Can you work these out from the model? Positions are in its coordinate system, mm. Face numbers are marked on the shaded views. A direction names the side the tool comes from. Round coordinates to 2 decimals unless told otherwise and drop trailing zeros. Order: outer loops, then holes, each group sorted by start corner. A loop starts at its lowest first (then second) coordinate and runs counter-clockwise, first axis right, second up. Notation, with made-up numbers: (-23.75, 17) -> (13.25, 17) arc R23 cw to (13.25, 49) -> close; hole circle Ø4 at (44, -23.75). An arc over 180 degrees is marked (long way). Use a Markdown table: item, result. Add a question column.
Q1. If we section it at A-A on y = 13: List the corners of the cut face in (x, z) for me, plus the area to 3 significant figures.
Q2. I need wall thicknesses on line 1 along X through (y, z) = (33, 6.8); line 2 along Y through (x, z) = (23, 7.05); line 3 along Y through (x, z) = (-11.5, 1.5). Which ranges of each line are inside material? Lowest first, please. Write a range as [from, to].
Q3. For the marked faces 1, 2 and 3, which set-ups out of +Z, -Z, +X, -X, +Y, -Y let a thin tool reach every point of the face, with its end or its side?
Q4. If we section it at B-B on x = -17: List the corners of the cut face in (y, z) for me.
Q5. I'm going to push flat-ended pins straight in: pin 1 Ø4.5 at (x, z) = (33.5, 2.5) entering from -Y; pin 2 Ø3 at (x, y) = (32, 8.5) entering from +Z; pin 3 Ø2 at (y, z) = (-32, 5.5) entering from -X; pin 4 Ø1 at (x, y) = (-10.5, -12) entering from +Z. Where does each tip first touch, or does it pass through?
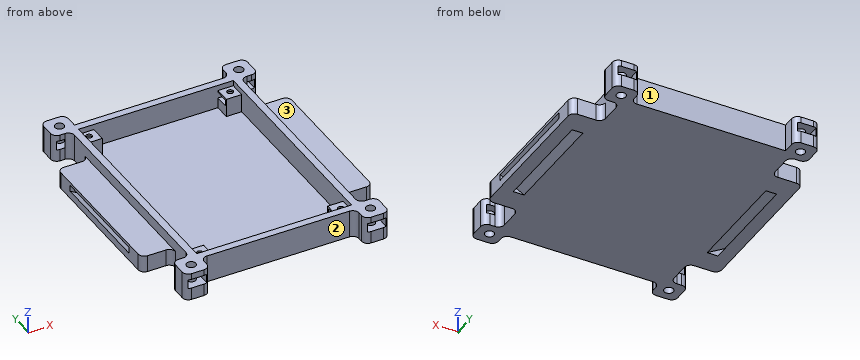
```python
from build123d import *

# Parameters (mm, degrees)
SKETCH_W        = 55.2
SKETCH_H        = 75.2
PAD_DEPTH       = 1.2
SKETCH001_W     = 55.2
SKETCH001_H     = 75.2
SKETCH001_R     = 1
PAD001_DEPTH    = 6
SKETCH002_W     = 55.2
SKETCH002_H     = 75.2
SKETCH002_W_2   = 50.4
SKETCH002_H_2   = 70.4
PAD002_DEPTH    = 1.8
SKETCH003_W     = 8
SKETCH003_H     = 8
PAD003_DEPTH    = 9
FILLET_R        = 2
SKETCH004_W     = 4.5
SKETCH004_H     = 2
POCKET_DEPTH    = 5
SKETCH006_R     = 1.5
POCKET001_DEPTH = 9.001
SKETCH007_W     = 6
SKETCH007_H     = 3
POCKET002_DEPTH = 8
SKETCH008_W     = 50
SKETCH008_H     = 5.5
PAD004_DEPTH    = 10
POCKET003_DEPTH = 17.5
FILLET001_R     = 2
SKETCH010_W     = 50
SKETCH010_H     = 5.5
PAD005_DEPTH    = 10
POCKET004_DEPTH = 17.5
FILLET002_R     = 2


with BuildPart() as part:
    # Sketch → Pad (new body)
    with BuildSketch(Plane.XY):
        Rectangle(SKETCH_W, SKETCH_H)
    extrude(amount=PAD_DEPTH)

    # Sketch001 (on Face6 of Pad) → Pad001 (join)
    with BuildSketch(Plane.XY.offset(1.2)):
        Rectangle(SKETCH001_W, SKETCH001_H)
        with Locations((-23, 33)):
            Circle(SKETCH001_R, mode=Mode.SUBTRACT)
        with Locations((23, 33)):
            Circle(SKETCH001_R, mode=Mode.SUBTRACT)
        with Locations((23, -33)):
            Circle(SKETCH001_R, mode=Mode.SUBTRACT)
        with Locations((-23, -33)):
            Circle(SKETCH001_R, mode=Mode.SUBTRACT)
        Polygon((-25.2, -30.2), (-25.2, 30.2), (-20.2, 30.2), (-20.2, 35.2), (20.2, 35.2), (20.2, 30.2), (25.2, 30.2), (25.2, -30.2), (20.2, -30.2), (20.2, -35.2), (-20.2, -35.2), (-20.2, -30.2), align=None, mode=Mode.SUBTRACT)
    extrude(amount=PAD001_DEPTH)

    # Sketch002 (on Face9 of Pad001) → Pad002 (join)
    with BuildSketch(Plane.XY.offset(7.2)):
        Rectangle(SKETCH002_W, SKETCH002_H)
        Rectangle(SKETCH002_W_2, SKETCH002_H_2, mode=Mode.SUBTRACT)
    extrude(amount=PAD002_DEPTH)

    # Sketch003 (on Face13 of Pad002) → Pad003 (join)
    with BuildSketch(Plane.XY.offset(9)):
        with Locations((29.2, -39.2)):
            Rectangle(SKETCH003_W, SKETCH003_H)
        with Locations((-29.2, -39.2)):
            Rectangle(SKETCH003_W, SKETCH003_H)
        with Locations((-29.2, 39.2)):
            Rectangle(SKETCH003_W, SKETCH003_H)
        with Locations((29.2, 39.2)):
            Rectangle(SKETCH003_W, SKETCH003_H)
    extrude(amount=-PAD003_DEPTH)

    # Fillet
    fillet_edges = [part.edges().sort_by_distance(p)[0] for p in [
        (25.2, -37.6, 4.2),
        (25.2, -37.6, 8.1),
        (25.2, -37.6, 0.6),
        (-33.2, 43.2, 4.5),
        (-25.2, 43.2, 4.5),
        (-33.2, 35.2, 4.5),
        (25.2, 37.6, 8.1),
        (25.2, 37.6, 4.2),
        (25.2, 37.6, 0.6),
        (25.2, 43.2, 4.5),
        (33.2, 43.2, 4.5),
        (33.2, 35.2, 4.5),
        (27.6, 35.2, 8.1),
        (27.6, 35.2, 4.2),
        (33.2, -35.2, 4.5),
        (27.6, -35.2, 4.2),
        (27.6, -35.2, 8.1),
        (27.6, -35.2, 0.6),
        (33.2, -43.2, 4.5),
        (25.2, -43.2, 4.5),
        (-25.2, -37.6, 8.1),
        (-25.2, -37.6, 4.2),
        (-25.2, -37.6, 0.6),
        (-25.2, -43.2, 4.5),
        (-33.2, -43.2, 4.5),
        (-33.2, -35.2, 4.5),
        (-27.6, -35.2, 4.2),
        (-27.6, -35.2, 8.1),
        (-27.6, -35.2, 0.6),
        (-27.6, 35.2, 8.1),
        (-27.6, 35.2, 4.2),
        (-27.6, 35.2, 0.6),
    ]]
    fillet(fillet_edges, radius=FILLET_R)

    # Sketch004 (on Face94 of Fillet) → Pocket (cut)
    with BuildSketch(Plane.YZ.offset(-20.2)):
        with Locations((32.95, 5.6)):
            Rectangle(SKETCH004_W, SKETCH004_H)
        with Locations((-32.95, 5.6)):
            Rectangle(SKETCH004_W, SKETCH004_H)
    pocket = extrude(amount=-POCKET_DEPTH, mode=Mode.SUBTRACT)

    # Mirrored: Pocket across YZ
    add(pocket.mirror(Plane.YZ), mode=Mode.SUBTRACT)

    # Sketch006 (on Face66 of Mirrored) → Pocket001 (cut, through all)
    with BuildSketch(Plane.XY.offset(9)):
        with Locations((-29.2, 39.2)):
            Circle(SKETCH006_R)
        with Locations((29.2, 39.2)):
            Circle(SKETCH006_R)
        with Locations((29.2, -39.2)):
            Circle(SKETCH006_R)
        with Locations((-29.2, -39.2)):
            Circle(SKETCH006_R)
    extrude(amount=-POCKET001_DEPTH, mode=Mode.SUBTRACT)

    # Sketch007 (on Face55 of Pocket001) → Pocket002 (cut)
    with BuildSketch(Plane.XZ.offset(43.2)):
        with Locations((-29.2, 5.5)):
            Rectangle(SKETCH007_W, SKETCH007_H)
        with Locations((29.2, 5.5)):
            Rectangle(SKETCH007_W, SKETCH007_H)
    pocket002 = extrude(amount=-POCKET002_DEPTH, mode=Mode.SUBTRACT)

    # Mirrored001: Pocket002 across XZ
    add(pocket002.mirror(Plane.XZ), mode=Mode.SUBTRACT)

    # Sketch008 (on Face45 of Mirrored001) → Pad004 (join)
    with BuildSketch(Plane(origin=(-27.6, 0, 0), x_dir=(0, -1, 0), z_dir=(-1, 0, 0))):
        with Locations((0, 2.75)):
            Rectangle(SKETCH008_W, SKETCH008_H)
    extrude(amount=PAD004_DEPTH)

    # Sketch009 → Pocket003 (cut, symmetric)
    with BuildSketch(Plane.XZ):
        Polygon((-37.6, 2.479274), (-33.305771, 0), (-29.805771, 0), (-37.6, 4.5), align=None)
    extrude(amount=POCKET003_DEPTH, both=True, mode=Mode.SUBTRACT)

    # Fillet001
    fillet001_edges = [part.edges().sort_by_distance(p)[0] for p in [
        (-27.6, 25, 3.35),
        (-27.6, 25, 0.6),
        (-27.6, -25, 3.35),
        (-27.6, -25, 0.6),
        (-37.6, -25, 2.75),
        (-37.6, 25, 2.75),
    ]]
    fillet(fillet001_edges, radius=FILLET001_R)

    # Sketch010 (on Face66 of Fillet001) → Pad005 (join)
    with BuildSketch(Plane.YZ.offset(27.6)):
        with Locations((0, 2.75)):
            Rectangle(SKETCH010_W, SKETCH010_H)
    extrude(amount=PAD005_DEPTH)

    # Sketch011 → Pocket004 (cut, symmetric)
    with BuildSketch(Plane.XZ):
        Polygon((37.6, 4.5), (29.805771, 0), (33.305771, 0), (37.6, 2.479274), align=None)
    extrude(amount=POCKET004_DEPTH, both=True, mode=Mode.SUBTRACT)

    # Fillet002
    fillet002_edges = [part.edges().sort_by_distance(p)[0] for p in [
        (37.6, 25, 2.75),
        (27.6, 25, 3.35),
        (27.6, 25, 0.6),
        (27.6, -25, 3.35),
        (27.6, -25, 0.6),
        (37.6, -25, 2.75),
    ]]
    fillet(fillet002_edges, radius=FILLET002_R)


solid = part.part
```
Answer below:
| question | item | result |
|---|---|---|
| 1 | outline | (-37.6, 0) -> (-33.31, 0) -> (-37.6, 2.48) -> close; (-37.6, 4.5) -> (-29.81, 0) -> (29.81, 0) -> (37.6, 4.5) -> (37.6, 5.5) -> (27.6, 5.5) -> (27.6, 9) -> (25.2, 9) -> (25.2, 1.2) -> (-25.2, 1.2) -> (-25.2, 9) -> (-27.6, 9) -> (-27.6, 5.5) -> (-37.6, 5.5) -> close; (33.31, 0) -> (37.6, 0) -> (37.6, 2.48) -> close |
| 1 | area | 189 mm² |
| 2 | line 1 | [-27.6, -24], [-22, -20.2], [20.2, 22], [24, 27.6] |
| 2 | line 2 | [-37.6, -34], [-32, -30.2], [30.2, 32], [34, 37.6] |
| 2 | line 3 | [-37.6, -35.2], [35.2, 37.6] |
| 3 | face 1 | +Z, -Z, +Y |
| 3 | face 2 | +Z, -Z, -Y |
| 3 | face 3 | +Z, +X |
| 4 | outline | (-37.6, 0) -> (37.6, 0) -> (37.6, 9) -> (35.2, 9) -> (35.2, 1.2) -> (-35.2, 1.2) -> (-35.2, 9) -> (-37.6, 9) -> close |
| 5 | pin 1 | y = -43.2 |
| 5 | pin 2 | z = 5.5 |
| 5 | pin 3 | x = -27.6 |
| 5 | pin 4 | z = 1.2 |
